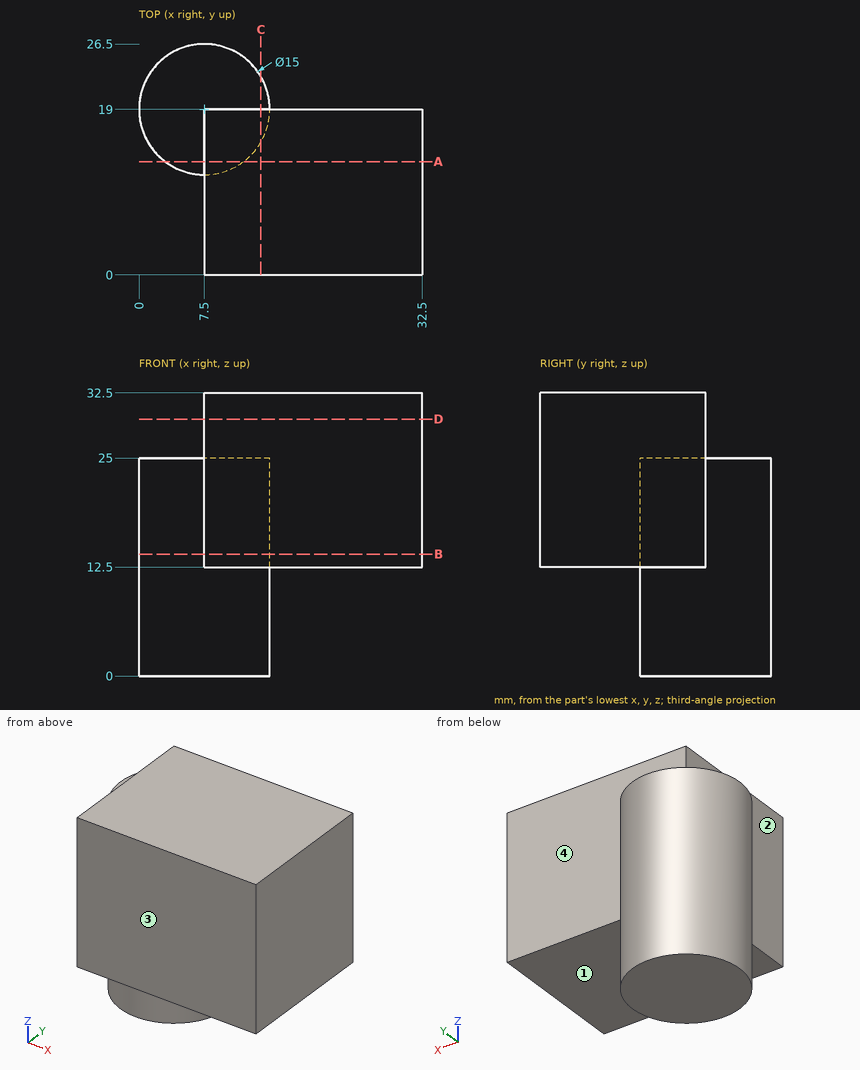
Job drawing, mm, ordinate dimensions from the low corner. One solid piece. A direction names the side the tool comes from. Coordinates: 2 decimals unless noted, no trailing zeros. Order: outer loops, then holes, each group sorted by start corner. A loop starts at its lowest first (then second) coordinate and runs counter-clockwise, first axis right, second up. Notation, with made-up numbers: (22, 66.25) -> (74, 66.25) arc R19 cw to (74, 91.25) -> close; hole circle Ø8 at (71.5, 14.25). An arc over 180 degrees is marked (long way). Return JSON: item names as keys, results as strings. Group by question number.
Item 1: Saw through at A-A on y = 13. Write the cut outline in (x, z).
Item 2: Saw through at D-D on z = 29.5. Write the cut outline in (x, y), then the cut area to 3 significant figures.
Item 3: Tool access for the marked faces 1, 2, 3 and 4: list every direction of +Z, -Z, +X, -X, +Y, -Y with a clear straight run to the whole face (end or side of a thin tool).
Item 4: Flat gauge pins, fed straight in: P1, Ø4, axis at x = 28, z = 27.5, coming from the +Y side; P2, Ø3, axis at y = 5.5, z = 16, coming from the -X side. Where does each tip first touch, or does it go through?
Item 5: Wall check: line 1 along Y through (x, z) = (21.5, 25); line 2 along X through (y, z) = (6.5, 27.5); line 3 along X through (y, z) = (19.25, 24). Give the ranges that are in metal, low to high. Write a range as [from, to].
Item 6: Saw through at C-C on x = 14. Write the cut outline in (y, z).
Item 7: Saw through at B-B on z = 14. Write the cut outline in (x, y).
Values found:
{
 "1": {"outline": "(3, 0) -> (12, 0) -> (12, 12.5) -> (32.5, 12.5) -> (32.5, 32.5) -> (7.5, 32.5) -> (7.5, 25) -> (3, 25) -> close"},
 "2": {"outline": "(7.5, 0) -> (32.5, 0) -> (32.5, 19) -> (7.5, 19) -> close", "area": "475 mm2"},
 "3": {"face 1": "-Z, +X, -Y", "face 2": "+Z, -X, -Y", "face 3": "+Z, -Z, +X, -X, -Y", "face 4": "+Z, +X, +Y"},
 "4": {"P1": "stops at y = 19", "P2": "stops at x = 7.5"},
 "5": {"line 1": "y = [0, 19]", "line 2": "x = [7.5, 32.5]", "line 3": "x = [0, 15]"},
 "6": {"outline": "(0, 12.5) -> (15.26, 12.5) -> (15.26, 0) -> (22.74, 0) -> (22.74, 25) -> (19, 25) -> (19, 32.5) -> (0, 32.5) -> close"},
 "7": {"outline": "(7.5, 0) -> (32.5, 0) -> (32.5, 19) -> (15, 19) arc R7.5 ccw (long way) to (7.5, 11.5) -> close"}
}
